from build123d import *

# Parameters (mm, degrees)
SKETCH1_R           = 1.25
BOSS_EXTRUDE2_DEPTH = 10
SKETCH3_R           = 2.5
CUT_EXTRUDE2_DEPTH  = 2


with BuildPart() as part:
    # Sketch1 → Boss-Extrude2 (new body)
    with BuildSketch(Plane(origin=(0, 0, 0), x_dir=(1, 0, 0), z_dir=(0, 1, 0))):
        Polygon((7.491574944, 45.496576397), (-56.267168264, 45.496576397), (-56.267168264, -33.972048376), (7.491574944, -33.906823563), align=None)
        with Locations(Location((-34.087168277, -18.903423613, 0), (0, 0, 270))):
            Circle(SKETCH1_R, mode=Mode.SUBTRACT)
        with Locations(Location((-13.887168277, -18.903423613, 0), (0, 0, 270))):
            Circle(SKETCH1_R, mode=Mode.SUBTRACT)
        with Locations(Location((-34.087168277, 30.496576397, 0), (0, 0, 270))):
            Circle(SKETCH1_R, mode=Mode.SUBTRACT)
        with Locations(Location((-13.887168277, 30.496576397, 0), (0, 0, 270))):
            Circle(SKETCH1_R, mode=Mode.SUBTRACT)
    extrude(amount=-BOSS_EXTRUDE2_DEPTH)

    # Sketch3 → Cut-Extrude2 (cut)
    with BuildSketch(Plane.XZ.offset(10)):
        with Locations(Location((-13.887168277, 18.903423613, 0), (0, 0, 270))):
            Circle(SKETCH3_R)
        with Locations(Location((-34.087168277, 18.903423613, 0), (0, 0, 270))):
            Circle(SKETCH3_R)
        with Locations(Location((-13.887168277, -30.496576397, 0), (0, 0, 270))):
            Circle(SKETCH3_R)
        with Locations(Location((-34.087168277, -30.496576397, 0), (0, 0, 270))):
            Circle(SKETCH3_R)
    extrude(amount=-CUT_EXTRUDE2_DEPTH, mode=Mode.SUBTRACT)


solid = part.part
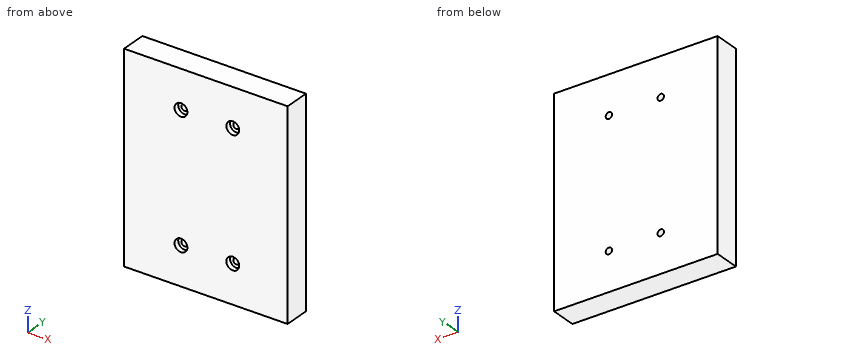
The listing builds one solid part. Answer for the finished solid, in the listing's coordinates (mm). Round coordinates to 2 decimals unless told otherwise and drop trailing zeros. Write each loop counter-clockwise with the first axis right and the second up, starting at its lowest first coordinate (ties: lowest second). Pieces come first, ordered by that corner, then holes. Notation, with made-up numbers: (64.25, -37.75) - (95.25, -37.75) arc R34 ccw to (95.25, -3.75) - close; hole circle Ø5 at (87, -16.5). An arc over 180 degrees is marked (long way). Use a Markdown table: item, result. Add a question column.
1. The part is cut by section B-B (y = -9). Write down the section's boundary in (x, z).
2. Consider line 1 (Z direction, x = -13.5, y = -1.5); line 2 (Z direction, x = -47.5, y = -6.25); line 3 (X direction, y = -5.25, z = 18.5). Determine where each line is inside the solid, lowest interval first.
3. The part is cut by section A-A (z = -30.5). Write down the section's boundary in (x, y).
4. Flat-ended cylindrical pins translate along their axes: P1, Ø4, axis at x = -34, z = 18.5, coming from the -Y side; P2, Ø6, axis at x = -34.09, z = 18.9, coming from the +Y side; P3, Ø1, axis at x = 0.5, y = -2, coming from the +Z side. Find the tip coordinate at first contact, or state that the pin passes through.
Reported:
| question | item | result |
|---|---|---|
| 1 | outline | (-56.27, -45.5) - (7.49, -45.5) - (7.49, 33.91) - (-56.27, 33.97) - close; hole circle Ø5 at (-34.09, -30.5); hole circle Ø5 at (-34.09, 18.9); hole circle Ø5 at (-13.89, -30.5); hole circle Ø5 at (-13.89, 18.9) |
| 2 | line 1 | -45.5 to -31.69, -29.31 to 17.71, 20.09 to 33.93 |
| 2 | line 2 | -45.5 to 33.96 |
| 2 | line 3 | -56.27 to -35.27, -32.9 to -15.07, -12.7 to 7.49 |
| 3 | outline | (-56.27, -10) - (-36.59, -10) - (-36.59, -8) - (-35.34, -8) - (-35.34, 0) - (-56.27, 0) - close; (-32.84, -8) - (-31.59, -8) - (-31.59, -10) - (-16.39, -10) - (-16.39, -8) - (-15.14, -8) - (-15.14, 0) - (-32.84, 0) - close; (-12.64, -8) - (-11.39, -8) - (-11.39, -10) - (7.49, -10) - (7.49, 0) - (-12.64, 0) - close |
| 4 | P1 | y = -8 |
| 4 | P2 | y = 0 |
| 4 | P3 | z = 33.91 |
